Design review of the part built by this model. Coordinates are the model's own, in mm. A direction names the side the tool comes from. Round coordinates to 2 decimals unless told otherwise and drop trailing zeros. Order: outer loops, then holes, each group sorted by start corner. A loop starts at its lowest first (then second) coordinate and runs counter-clockwise, first axis right, second up. Notation, with made-up numbers: (71.5, 36.25) - (129.5, 36.25) arc R20 cw to (129.5, 51.25) - close; hole circle Ø3 at (14, -33). An arc over 180 degrees is marked (long way). Write item = value, one per line.
from build123d import *

# Parameters (mm, degrees)
EXTRUDE_1_DEPTH     = 48
HOLE_WIZARD_M8_1_D  = 6.8
SKETCH_4_W          = 4
SKETCH_4_H          = 18
CUT_EXTRUDE_1_DEPTH = 63.136945532


with BuildPart() as part:
    # 草图1 → 凸台-拉伸1 (new, symmetric)
    with BuildSketch(Plane(origin=(0, 0, 0), x_dir=(0, 0, -1), z_dir=(1, 0, 0))):
        Polygon((0, 0), (39, 0), (24, 6), (0, 6), align=None)
    extrude(amount=EXTRUDE_1_DEPTH, both=True)

    # M8 螺纹孔1 (through all)
    with Locations(Plane(origin=(0, 6, 0), x_dir=(1, 0, 0), z_dir=(0, 1, 0))):
        with Locations((32.5, 12), (-32.5, 12)):
            Hole(HOLE_WIZARD_M8_1_D / 2)

    # 草图4 → 切除-拉伸-薄壁1 (cut, symmetric)
    with BuildSketch(Plane(origin=(0, 6, 0), x_dir=(1, 0, 0), z_dir=(0, 1, 0))):
        with Locations((-31, 30)):
            Rectangle(SKETCH_4_W, SKETCH_4_H)
    cut_extrude_1 = extrude(amount=CUT_EXTRUDE_1_DEPTH, both=True, mode=Mode.SUBTRACT)

    # 镜向1: 切除-拉伸-薄壁1 across plane
    add(cut_extrude_1.mirror(Plane(origin=(0, 0, 0), x_dir=(0, 0, 1), z_dir=(1, 0, 0))), mode=Mode.SUBTRACT)


solid = part.part
1) To check wall thickness, follow L1, parallel to X at y = 1.95, z = -12; L2, parallel to X at y = 4.25, z = -24.5; L3, parallel to Z at x = -32.5, y = 2.5. State the ranges of each line that lie inside material, in increasing order. Write a range as from..to.
Findings:
L1 = -48..-35.9, -29.1..29.1, 35.9..48
L2 = -48..-33, -29..29, 33..48
L3 = -21..-15.4, -8.6..0
2) The part is to be moulded in two halves that separate along Z. For faces 1 (the cylindrical face through (-34.1, 3, -9)), 2 (the flat face through (1, 6, -12)), 3 (the flat face through (-40.39, 2.96, -31.6)), say which applies: released by +Z, released by -Z, zero draft, split by the parting line, or undercut.
Findings:
face_1 = undercut
face_2 = zero draft
face_3 = released by -Z
3) We need section B-B on y = 3.5. Write out the cut boundary in (x, z), and give its area (3 significant figures).
Findings:
outline = (-48, -30.25) - (-33, -30.25) - (-33, -21) - (-29, -21) - (-29, -30.25) - (29, -30.25) - (29, -21) - (33, -21) - (33, -30.25) - (48, -30.25) - (48, 0) - (-48, 0) - close; hole circle Ø6.8 at (-32.5, -12); hole circle Ø6.8 at (32.5, -12)
area = 2,760 mm^2
4) We need section D-D on x = -38. Write out the cut boundary in (y, z).
Findings:
outline = (0, -39) - (6, -24) - (6, 0) - (0, 0) - close
5) We need section A-A on z = -28. Write out the cut boundary in (x, y), and give its area (3 significant figures).
Findings:
outline = (-48, 0) - (-33, 0) - (-33, 4.4) - (-48, 4.4) - close; (-29, 0) - (29, 0) - (29, 4.4) - (-29, 4.4) - close; (33, 0) - (48, 0) - (48, 4.4) - (33, 4.4) - close
area = 387 mm^2
6) For faces 4 (the flat face through (1, 0, -19)), 5 (the flat face through (-31, 3, -21)), list the 3-axis set-ups (+Z, -Z, +X, -X, +Y, -Y) from which the entire face can be reached by the end or side of a thin tool; tool diameter is ignored.
Findings:
face_4 = +Z, -Z, +X, -X, -Y
face_5 = -Z, +Y, -Y
7) We need section C-C on z = -34. Write out the cut boundary in (x, y), and give its area (3 significant figures).
Findings:
outline = (-48, 0) - (-33, 0) - (-33, 2) - (-48, 2) - close; (-29, 0) - (29, 0) - (29, 2) - (-29, 2) - close; (33, 0) - (48, 0) - (48, 2) - (33, 2) - close
area = 176 mm^2
8) Clearance check with a flat-ended pin moving along its axis: pin 1 Ø1.2 at (x, y) = (-32, 2.5) entering from -Z. State where the tip first meets the part, or that it passes through.
Findings:
pin_1 = -21
